Work out the finished part from the listing and answer in its coordinate system (mm). A direction names the side the tool comes from. Coordinates: 2 decimals unless noted, no trailing zeros. Loops run counter-clockwise (first coordinate to the right, second up) from the corner with the lowest first, then second, coordinate; pieces in that order, holes last. Notation, with made-up numbers: (12, 7) - (37, 7) arc R11 cw to (37, 12) - close; hole circle Ø2 at (58, 12). An arc over 180 degrees is marked (long way). Write each question's results on one line, items separated by ' | '. Start each with the question number.
Item 1: For a pull along Y with two mould halves and no side action, classify faces 3 (the face through (52, 1, 76.2)), 4 (the face through (-46.108, 30.518, 1.067)), 5 (the face through (39.72, 88.71, 0.89)) as +Y half, -Y half, draft (parallel to the pull), parting line (faces both ways), or undercut.
Item 2: Consider probe 1 along Z at (x, y) = (86, 45); probe 2 along X at (y, z) = (56.5, 2); probe 3 along X at (y, z) = (-30.5, 46.5). Determine where each line is inside the solid, lowest interval first. Write a range as [from, to].
Item 3: Section A-A, the plane y = 0 is taken. Write down the section's boundary in (x, z).
Item 4: Each of these flat-tipped pins is pushed along its axis until it touches: pin 1 Ø6 at (x, y) = (129.5, 66.5) entering from -Z; pin 2 Ø1.5 at (x, z) = (129.5, 25.5) entering from -Y; pin 3 Ø4 at (x, z) = (71, 61) entering from -Y; pin 4 Ø1.5 at (y, z) = (22, 9.5) entering from -X. Where does it stop, or does it pass through?
Item 5: Section C-C, the plane z = 32 is taken. Write down the section's boundary in (x, y), plus the area to 3 significant figures.
Item 6: A tool of negligible diameter and unlimited length cuts with its end or side. For faces 1 (the face through (50, 1, 63.5)), 2 (the face through (52, 1, -76.2)), from which of +Z, -Z, +X, -X, +Y, -Y can it reach the whole face along a straight path? Write none if from no direction.
Item 7: Section B-B, the plane x = -22.5 is taken. Write down the section's boundary in (y, z), plus the area to 3 significant figures.
from build123d import *

# Parameters (mm, degrees)
F0_W     = 101.6
F0_H     = 152.4
F2_T     = -12.7
F3_R     = 89.4707101345
F4_DEPTH = 63.5


with BuildPart() as f1:
    # F0 (on Front) → F1 (revolve)
    with BuildSketch(Plane.XZ):
        Rectangle(F0_W, F0_H)
    revolve(axis=Axis((50.8, 0, 0), (0, 0, -1)))

    # F2 (hollow: no face is removed)
    offset(amount=F2_T, mode=Mode.SUBTRACT)

    # F3 (on Top) → F4 (cut, symmetric)
    with BuildSketch(Plane.XY):
        with Locations((51.3707101345, 0)):
            Circle(F3_R)
    extrude(amount=F4_DEPTH, both=True, mode=Mode.SUBTRACT)


solid = f1.part
Answer key:
1) face 3: draft | face 4: parting line | face 5: undercut
2) probe 1: z = [-76.2, -63.5], [63.5, 76.2] | probe 2: x = [-33.64, -18], [120.74, 135.24] | probe 3: x = [-46.11, -32.74], [135.48, 147.71]
3) outline: (-50.8, -76.2) - (152.4, -76.2) - (152.4, 76.2) - (-50.8, 76.2) - close; hole (-38.1, -63.5) - (140.84, -63.5) - (140.84, 63.5) - (-38.1, 63.5) - close
4) pin 1: stops at z = -76.2 | pin 2: stops at y = -65.16 | pin 3: stops at y = -99.96 | pin 4: stops at x = -48.55
5) outline: circle Ø203.2 at (50.8, 0); hole circle Ø178.94 at (51.37, 0) | area: 7,280 mm^2
6) face 1: none | face 2: -Z, +X, -X, +Y, -Y
7) outline: (-70.35, -76.2) - (70.35, -76.2) - (70.35, 76.2) - (-70.35, 76.2) - close; hole (-50.48, -63.5) - (50.48, -63.5) - (50.48, 63.5) - (-50.48, 63.5) - close | area: 8,620 mm^2
